Geometry check sheet. Reference: the model listing, model coordinates, mm. Face numbers are marked on the shaded views. Round coordinates to 2 decimals unless told otherwise and drop trailing zeros. Order: outer loops, then holes, each group sorted by start corner. A loop starts at its lowest first (then second) coordinate and runs counter-clockwise, first axis right, second up. Notation, with made-up numbers: M 35.5,10 L 74.5,10 A34 cw 74.5,48 Z; hole C 5.5,35.5 d6. An arc over 180 degrees is marked long. Answer as a JSON object with one key per item and string values. Group by question number.
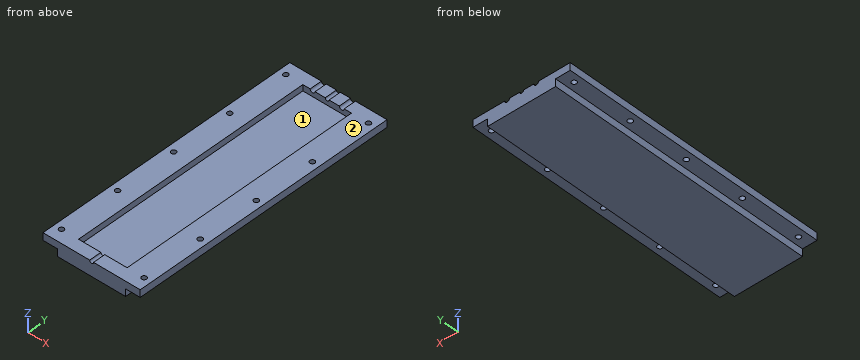
```python
from build123d import *

# Parameters (mm, degrees)
SKETCH1_W           = 28
SKETCH1_H           = 6
BOSS_EXTRUDE1_DEPTH = 105
SKETCH2_W           = 20
SKETCH2_H           = 5
CUT_EXTRUDE1_DEPTH  = 100
SKETCH3_W           = 6
SKETCH3_H           = 3
BOSS_EXTRUDE2_DEPTH = 105
SKETCH6_R           = 0.8
CUT_EXTRUDE4_DEPTH  = 10
BOSS_EXTRUDE3_DEPTH = 5
SKETCH7_R           = 1
CUT_EXTRUDE5_DEPTH  = 10
SKETCH9_R           = 1
CUT_EXTRUDE6_DEPTH  = 5


with BuildPart() as part:
    # Sketch1 → Boss-Extrude1 (new body)
    with BuildSketch(Plane(origin=(0, 0, 0), x_dir=(1, 0, 0), z_dir=(0, 1, 0))):
        with Locations((0, 3)):
            Rectangle(SKETCH1_W, SKETCH1_H)
    extrude(amount=BOSS_EXTRUDE1_DEPTH)

    # Sketch2 → Cut-Extrude1 (cut)
    with BuildSketch(Plane(origin=(0, 105, 0), x_dir=(1, 0, 0), z_dir=(0, 1, 0))):
        Rectangle(SKETCH2_W, SKETCH2_H)
    extrude(amount=-CUT_EXTRUDE1_DEPTH, mode=Mode.SUBTRACT)

    # Sketch3 → Boss-Extrude2 (add)
    with BuildSketch(Plane(origin=(0, 105, 0), x_dir=(1, 0, 0), z_dir=(0, 1, 0))):
        with Locations((17, 1.5)):
            Rectangle(SKETCH3_W, SKETCH3_H)
        with Locations((-17, 1.5)):
            Rectangle(SKETCH3_W, SKETCH3_H)
    extrude(amount=-BOSS_EXTRUDE2_DEPTH)

    # Sketch6 → Cut-Extrude4 (cut)
    with BuildSketch(Plane.XZ):
        Circle(SKETCH6_R)
    extrude(amount=-CUT_EXTRUDE4_DEPTH, mode=Mode.SUBTRACT)

    # Sketch8 → Boss-Extrude3 (add)
    with BuildSketch(Plane(origin=(0, 105, 0), x_dir=(1, 0, 0), z_dir=(0, 1, 0))):
        with BuildLine():
            Line((-0.8, 0), (-10, 0))
            Line((-10, 0), (-20, 0))
            Line((-20, 0), (-20, 3))
            Line((-20, 3), (-14, 3))
            Line((-14, 3), (-14, 6))
            Line((-14, 6), (14, 6))
            Line((14, 6), (14, 3))
            Line((14, 3), (20, 3))
            Line((20, 3), (20, 0))
            Line((20, 0), (10, 0))
            Line((10, 0), (0.8, 0))
            ThreePointArc((0.8, 0), (0, 0.8), (-0.8, 0))
        make_face()
    extrude(amount=BOSS_EXTRUDE3_DEPTH)

    # Sketch7 → Cut-Extrude5 (cut)
    with BuildSketch(Plane(origin=(0, 0, -3), x_dir=(-1, 0, 0), z_dir=(0, 0, -1))):
        with Locations((-17, 5)):
            Circle(SKETCH7_R)
        with Locations((-17, 30)):
            Circle(SKETCH7_R)
        with Locations((-17, 55)):
            Circle(SKETCH7_R)
        with Locations((-17, 80)):
            Circle(SKETCH7_R)
        with Locations((17, 80)):
            Circle(SKETCH7_R)
        with Locations((17, 55)):
            Circle(SKETCH7_R)
        with Locations((17, 30)):
            Circle(SKETCH7_R)
        with Locations((17, 5)):
            Circle(SKETCH7_R)
        with Locations((-17, 105)):
            Circle(SKETCH7_R)
        with Locations((17, 105)):
            Circle(SKETCH7_R)
    extrude(amount=-CUT_EXTRUDE5_DEPTH, mode=Mode.SUBTRACT)

    # Sketch9 → Cut-Extrude6 (cut)
    with BuildSketch(Plane(origin=(0, 110, 0), x_dir=(1, 0, 0), z_dir=(0, 1, 0))):
        with Locations((6, 0)):
            Circle(SKETCH9_R)
        with Locations((-6, 0)):
            Circle(SKETCH9_R)
    extrude(amount=-CUT_EXTRUDE6_DEPTH, mode=Mode.SUBTRACT)


solid = part.part
```
1) Sectioned sample at C-C (x = 6). Record the boundary of the cut face in (y, z).
2) Thickness scan on line 1 along Y through (x, z) = (17, -0.65); line 2 along X through (y, z) = (64.5, -2.25); line 3 along X through (y, z) = (42, -5). Record the ranges inside material, lowest first. Write a range as [from, to].
3) Release check for a two-part mould opening along X. For the marked faces 1 and 2 record: +X half, -X half, draft (parallel to the pull), parting line (faces both ways), or undercut.
4) Go/stop test with flat-tipped pins: P1, Ø2, axis at x = -6.5, y = 42, coming from the +Z side; P2, Ø2.5, axis at y = 43, z = -4.5, coming from the -X side; P3, Ø6.5, axis at x = -17.5, y = 79.5, coming from the -Z side. Record where each tip stops, or that it passes through.
5) Sectioned sample at D-D (y = 75.5). Record the boundary of the cut face in (x, z), then the cut area to 3 significant figures.
6) Sectioned sample at A-A (x = -17). Record the boundary of the cut face in (y, z), then the cut area to 3 significant figures.
7) Sectioned sample at B-B (y = 55). Record the boundary of the cut face in (x, z).
Final values:
{
 "1": {"outline": "M 0,-6 L 110,-6 L 110,-1 L 105,-1 L 105,-2.5 L 5,-2.5 L 5,0 L 0,0 Z"},
 "2": {"line 1": "y = [0, 4], [6, 29], [31, 54], [56, 79], [81, 104], [106, 110]", "line 2": "x = [-20, -10], [10, 20]", "line 3": "x = [-14, 14]"},
 "3": {"face 1": "undercut", "face 2": "draft"},
 "4": {"P1": "stops at z = -2.5", "P2": "stops at x = -14", "P3": "stops at z = -3"},
 "5": {"outline": "M -20,-3 L -14,-3 L -14,-6 L 14,-6 L 14,-3 L 20,-3 L 20,0 L 10,0 L 10,-2.5 L -10,-2.5 L -10,0 L -20,0 Z", "area": "154 mm^2"},
 "6": {"outline": "M 0,-3 L 4,-3 L 4,0 L 0,0 Z; M 6,-3 L 29,-3 L 29,0 L 6,0 Z; M 31,-3 L 54,-3 L 54,0 L 31,0 Z; M 56,-3 L 79,-3 L 79,0 L 56,0 Z; M 81,-3 L 104,-3 L 104,0 L 81,0 Z; M 106,-3 L 110,-3 L 110,0 L 106,0 Z", "area": "300 mm^2"},
 "7": {"outline": "M -20,-3 L -18,-3 L -18,0 L -20,0 Z; M -16,-3 L -14,-3 L -14,-6 L 14,-6 L 14,-3 L 16,-3 L 16,0 L 10,0 L 10,-2.5 L -10,-2.5 L -10,0 L -16,0 Z; M 18,-3 L 20,-3 L 20,0 L 18,0 Z"}
}
